Answer from the drawing. Dimensions are ordinates in mm from the lowest x, y and z of the part. Give positions to 0.01 mm unless a question says otherwise; leave off trailing zeros. Loops run counter-clockwise (first coordinate to the right, second up) from the corner with the lowest first, then second, coordinate; pieces in that order, holes last. Notation, with made-up numbers: (32, -12) -> (81, -12) arc R16 cw to (81, 16) -> close; hole circle Ø1 at (62.25, 79.25). An arc over 180 degrees is marked (long way). Return JSON: item names as keys, results as strings. Group by question number.
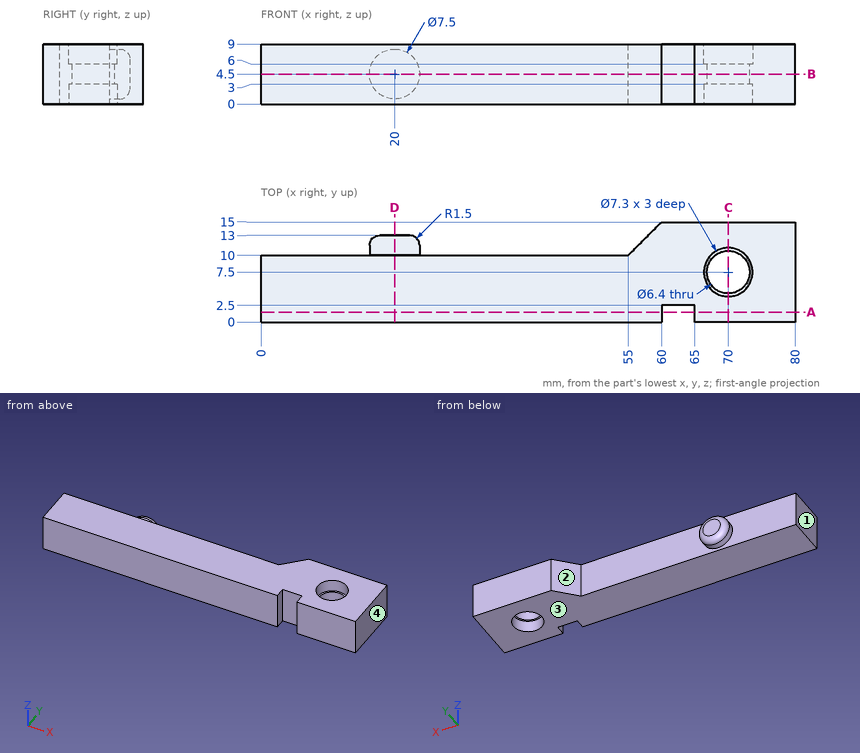
1. Straight lines are drawn through the part: line 1 (Y direction, x = 70, z = 2.2); line 2 (X direction, y = 1.5, z = 3.25); line 3 (X direction, y = 7.5, z = 3.85). For each, find the intervals that lie inside material, in ascending order. Write a range as from..to.
2. Section B-B on z = 4.5 is taken. Determine the outline of the cut face in (x, y), then the cut area to 3 significant figures.
3. Section C-C on x = 70 is taken. Determine the outline of the cut face in (y, z), then the cut area to 3 significant figures.
4. Flat-ended cylindrical pins translate along their axes: pin 1 Ø1.3 at (x, z) = (19.5, 4) entering from +Y; pin 2 Ø5 at (x, z) = (53.5, 5) entering from +Y; pin 3 Ø3 at (x, z) = (24, 8) entering from +Y. Find the tip coordinate at first contact, or state that the pin passes through.
5. Section A-A on y = 1.5 is taken. Determine the outline of the cut face in (x, z).
6. Section D-D on x = 20 is taken. Determine the outline of the cut face in (y, z).
7. Determine the mould class of the marked faces 1, 2, 3 and 4 for opening direction X: pulls with the +X half, pulls with the -X half, needs draft (parallel to the pull), parting line crosses it, or undercut.
Completed:
{
 "1": {"line 1": "y = 0..3.85, 11.15..15", "line 2": "x = 0..60, 65..80", "line 3": "x = 0..66.8, 73.2..80"},
 "2": {"outline": "(0, 0) -> (60, 0) -> (60, 2.5) -> (65, 2.5) -> (65, 0) -> (80, 0) -> (80, 15) -> (60, 15) -> (55, 10) -> (23.75, 10) -> (23.75, 11.5) arc R1.5 ccw to (22.25, 13) -> (17.75, 13) arc R1.5 ccw to (16.25, 11.5) -> (16.25, 10) -> (0, 10) -> close; hole circle Ø6.4 at (70, 7.5)", "area": "889 mm²"},
 "3": {"outline": "(0, 0) -> (3.85, 0) -> (3.85, 3) -> (4.3, 3) -> (4.3, 6) -> (3.85, 6) -> (3.85, 9) -> (0, 9) -> close; (10.7, 3) -> (11.15, 3) -> (11.15, 0) -> (15, 0) -> (15, 9) -> (11.15, 9) -> (11.15, 6) -> (10.7, 6) -> close", "area": "72.0 mm²"},
 "4": {"pin 1": "stops at y = 13", "pin 2": "stops at y = 11", "pin 3": "stops at y = 10"},
 "5": {"outline": "(0, 0) -> (60, 0) -> (60, 9) -> (0, 9) -> close; (65, 0) -> (80, 0) -> (80, 9) -> (65, 9) -> close"},
 "6": {"outline": "(0, 0) -> (10, 0) -> (10, 0.75) -> (11.5, 0.75) arc R1.5 ccw to (13, 2.25) -> (13, 6.75) arc R1.5 ccw to (11.5, 8.25) -> (10, 8.25) -> (10, 9) -> (0, 9) -> close"},
 "7": {"face 1": "pulls with the -X half", "face 2": "undercut", "face 3": "needs draft", "face 4": "pulls with the +X half"}
}
